Could you check a few things on this model? Use its own coordinates, in mm. A direction names the side the tool comes from. Give positions to 0.01 mm unless a question says otherwise; leave off trailing zeros. Write each loop counter-clockwise with the first axis right and the second up, starting at its lowest first coordinate (ties: lowest second). Pieces come first, ordered by that corner, then holes. Notation, with made-up numbers: (-13.5, 51) - (11.5, 51) arc R21 cw to (11.5, 71) - close; hole circle Ø8 at (39.5, -16.75). An arc over 180 degrees is marked (long way). Answer in a Markdown table with one row per item.
from build123d import *

# Parameters (mm, degrees)
BOSS_EXTRUDE1_DEPTH = 12.7
SHELL1_T            = 5.08
SKETCH1_3_R         = 1.651
SKETCH1_3_R_2       = 1.6509999999999996
CUT_EXTRUDE1_DEPTH  = 12.192
SKETCH2_R           = 24.765
CUT_EXTRUDE2_DEPTH  = 5.08


with BuildPart() as part:
    # Sketch1 → Boss-Extrude1 (new body)
    with BuildSketch(Plane(origin=(0, 0, 0), x_dir=(1, 0, 0), z_dir=(0, 1, 0))):
        with BuildLine():
            ThreePointArc((25.18661681826276, 14.541500000000127), (14.541499999999942, 25.186616818262866), (1.78e-15, 29.083000000000002))
            Line((0, 29.083000000000002), (0, 24.384))
            ThreePointArc((-2.409e-14, 24.384), (1.1674332957389815, 23.900433295739), (1.651, 22.733))
            ThreePointArc((1.651, 22.733), (1.1674332957389804, 21.565566704261002), (-2.523e-14, 21.082))
            Line((0, 21.082), (0, 16.383))
            ThreePointArc((1e-15, 16.383000000000003), (8.191499999999966, 14.188094190200482), (14.188094190200419, 8.191500000000074))
            Line((14.188094190200417, 8.191500000000072), (18.257547562583486, 10.541000000000096))
            ThreePointArc((18.257547562583472, 10.541000000000121), (18.86185550423157, 12.796307941648193), (21.11716344587966, 12.192000000000167))
            Line((21.117163445879694, 12.19200000000011), (25.18661681826275, 14.541500000000124))
        make_face()
        with BuildLine():
            ThreePointArc((1.651, 22.733), (1.1674332957389815, 23.900433295739), (-2.409e-14, 24.384))
            Line((0, 24.384), (0, 21.082))
            ThreePointArc((-2.523e-14, 21.082), (1.1674332957389804, 21.565566704261002), (1.651, 22.733))
        make_face()
        with BuildLine():
            Line((0, 21.082), (0, 24.384))
            ThreePointArc((-2.409e-14, 24.384), (-1.651, 22.733), (-2.523e-14, 21.082))
        make_face()
        with BuildLine():
            Line((0, 24.384), (0, 29.083000000000002))
            ThreePointArc((1.78e-15, 29.083000000000002), (-2.5347504663301574, 28.972330404602236), (-5.050209951087366, 28.641163880854045))
            Line((-5.050209951087367, 28.641163880854048), (-2.8448780947173375, 16.134105417599))
            ThreePointArc((-2.8448780947173375, 16.134105417599006), (-1.4278725334348923, 16.320657738837067), (1e-15, 16.383000000000003))
            Line((0, 16.383), (0, 21.082))
            ThreePointArc((-2.523e-14, 21.082), (-1.651, 22.733), (-2.409e-14, 24.384))
        make_face()
        with BuildLine():
            ThreePointArc((21.338355504231593, 11.366500000000098), (21.282099043434833, 11.793810243464398), (21.11716344587966, 12.192000000000167))
            Line((21.117163445879694, 12.19200000000011), (18.257547562583486, 10.541000000000096))
            ThreePointArc((18.257547562583472, 10.541000000000121), (20.11466574769584, 9.771756460796842), (21.338355504231593, 11.366500000000098))
        make_face()
        with BuildLine():
            Line((18.257547562583486, 10.541000000000096), (21.117163445879694, 12.19200000000011))
            ThreePointArc((21.11716344587966, 12.192000000000167), (18.86185550423157, 12.796307941648193), (18.257547562583472, 10.541000000000121))
        make_face()
        with BuildLine():
            ThreePointArc((27.32908049031651, 9.9469718283406), (26.358149370386823, 12.291006906204913), (25.18661681826276, 14.541500000000127))
            Line((25.18661681826275, 14.541500000000124), (21.117163445879694, 12.19200000000011))
            ThreePointArc((21.11716344587966, 12.192000000000167), (21.282099043434833, 11.793810243464398), (21.338355504231593, 11.366500000000098))
            ThreePointArc((21.338355504231593, 11.366500000000098), (20.11466574769584, 9.771756460796842), (18.257547562583472, 10.541000000000121))
            Line((18.257547562583486, 10.541000000000096), (14.188094190200417, 8.191500000000072))
            ThreePointArc((14.188094190200419, 8.191500000000074), (14.848040475021392, 6.923754982097979), (15.394984206335495, 5.603316008104555))
            Line((15.394984206335494, 5.603316008104554), (27.329080490316503, 9.946971828340597))
        make_face()
    extrude(amount=BOSS_EXTRUDE1_DEPTH)

    # Shell1
    shell1_openings = [part.faces().sort_by_distance(p)[0] for p in [
        (21.362032348, 6.35, -7.775143918),
        (8.1915, 6.35, -14.18809419),
        (-3.947544023, 6.35, -22.387634649),
    ]]
    offset(amount=SHELL1_T, openings=shell1_openings, kind=Kind.INTERSECTION)

    # Sketch1<3> → Cut-Extrude1 (cut)
    with BuildSketch(Plane(origin=(0, 0, 0), x_dir=(1, 0, 0), z_dir=(0, 1, 0))):
        with Locations(Location((0, 22.733, 0), (0, 0, 270))):
            Circle(SKETCH1_3_R)
        with Locations(Location((19.687355504231594, 11.366500000000098, 0), (0, 0, 270))):
            Circle(SKETCH1_3_R_2)
    extrude(amount=-CUT_EXTRUDE1_DEPTH, mode=Mode.SUBTRACT)

    # Sketch2 → Cut-Extrude2 (cut)
    with BuildSketch(Plane(origin=(0, 17.78, 0), x_dir=(1, 0, 0), z_dir=(0, 1, 0))):
        Circle(SKETCH2_R)
    extrude(amount=-CUT_EXTRUDE2_DEPTH, mode=Mode.SUBTRACT)


solid = part.part
1) If I drill on line 1 (Y direction, x = 23, z = -16); line 2 (Z direction, x = 0, y = 12.25); line 3 (Y direction, x = 12.5, z = -14), over which ranges is the centre line in solid material (lowest first)?
Check values:
| item | result |
|---|---|
| line 1 | y = -5.08 to 0, 12.7 to 17.78 |
| line 2 | z = -34.16 to -29.08 |
| line 3 | y = -5.08 to 0 |
2) Imagine slicing it at A-A (x = 0). List the corners of the cut face in (y, z) for me (3 decimals).
Check values:
| item | result |
|---|---|
| outline | (-5.08, -34.163) - (17.78, -34.163) - (17.78, -24.765) - (12.7, -24.765) - (12.7, -29.083) - (0, -29.083) - (0, -24.384) - (-5.08, -24.384) - close; (-5.08, -21.082) - (0, -21.082) - (0, -16.383) - (-5.08, -16.383) - close |
3) Imagine slicing it at D-D (x = 24.5). List the corners of the cut face in (y, z) for me, then the cut area to 3 significant figures.
Check values:
| item | result |
|---|---|
| outline | (-5.08, -23.81) - (17.78, -23.81) - (17.78, -8.92) - (12.7, -8.92) - (12.7, -15.67) - (0, -15.67) - (0, -8.92) - (-5.08, -8.92) - close |
| area | 255 mm2 |
4) Imagine slicing it at B-B (x = 7). List the corners of the cut face in (y, z) for me, then the cut area to 3 significant figures.
Check values:
| item | result |
|---|---|
| outline | (-5.08, -33.44) - (17.78, -33.44) - (17.78, -23.76) - (12.7, -23.76) - (12.7, -28.23) - (0, -28.23) - (0, -14.81) - (-5.08, -14.81) - close |
| area | 210 mm2 |
5) On a 3-axis mill with a long thin cutter (end or side, diameter ignored), from which of +Z, -Z, +X, -X, +Y, -Y can I reach the whole of each face in a straight line? I mean faces 1 (the face through (18.076, -2.504, -11.724)), 2 (the face through (14.79, 6.26, -25.04)). Say none if no direction works.
Check values:
| item | result |
|---|---|
| face 1 | +Y, -Y |
| face 2 | +Z |
6) Imagine slicing it at C-C (y = 6.5). List the corners of the cut face in (x, z) for me, then the cut area to 3 significant figures.
Check values:
| item | result |
|---|---|
| outline | (-5.93, -33.64) arc R34.16 ccw to (32.1, -11.68) - (27.33, -9.95) arc R29.08 cw to (-5.05, -28.64) - close |
| area | 224 mm2 |
7) We'd pull the mould along X, two halves only. Please class faces 3 (the face through (29.2, 3.65, -10.63)), 4 (the face through (13, 17.78, -24)), 5 (the face through (12.592, 15.276, -21.325)): +X half, -X half, draft (parallel to the pull), parting line (faces both ways), or undercut.
Check values:
| item | result |
|---|---|
| face 3 | +X half |
| face 4 | draft |
| face 5 | undercut |
8) Will these pins go through, and if not, where does the flat tip stop? P1, Ø12, axis at x = 25.5, y = -2.5, coming from the -Z side; P2, Ø5, axis at x = 6.5, y = -0.5, coming from the -Z side; P3, Ø10, axis at x = 4.5, z = -14.5, coming from the +Y side.
Check values:
| item | result |
|---|---|
| P1 | stops at z = -28.05 |
| P2 | stops at z = -33.93 |
| P3 | stops at y = 0 |
